Here's how the part is built. I have some questions about the finished solid (model axes, mm). A direction names the side the tool comes from. Round coordinates to 2 decimals unless told otherwise and drop trailing zeros. Loops run counter-clockwise (first coordinate to the right, second up) from the corner with the lowest first, then second, coordinate; pieces in that order, holes last. Notation, with made-up numbers: (82, 3.5) -> (141, 3.5) arc R29 ccw to (141, 36.5) -> close; hole circle Ø3 at (-39.75, 34). An arc over 180 degrees is marked (long way). Use CSV: the item, a comma, the result in double quotes. Start each with the question number.
Autodesk Inventor part; units mm, degrees
ref_plane "YZ Plane" through (0, 0, 0) normal (1, 0, 0) x (0, 1, 0)
ref_plane "XZ Plane" through (0, 0, 0) normal (0, 1, 0) x (-1, 0, 0)
ref_plane "XY Plane" through (0, 0, 0) normal (0, 0, 1) x (1, 0, 0)
sketch "Sketch1" plane through (0, 0, 0) normal (0, 0, 1) x (1, 0, 0)
  line L0 (-95, -10) -> (95, -10)
  line L1 (95, -10) -> (95, 10)
  line L2 (95, 10) -> (-95, 10)
  line L3 (-95, 10) -> (-95, -10)
  line L4 (-95, -10) -> (95, 10) construction
  line L5 (95, -10) -> (-95, 10) construction
  line L6 (-133, 0) -> (133, 0) construction
  line L7 (-83, -5.5) -> (-6, -5.5)
  line L8 (-6, -5.5) -> (-6, 5.5)
  line L9 (-6, 5.5) -> (-83, 5.5)
  line L10 (-83, 5.5) -> (-83, -5.5)
  line L11 (-83, -5.5) -> (-6, 5.5) construction
  line L12 (-6, -5.5) -> (-83, 5.5) construction
  line L13 (0, 14.2899) -> (0, -14.2899) construction
  line L14 (83, -5.5) -> (6, -5.5)
  line L15 (6, -5.5) -> (6, 5.5)
  line L16 (6, 5.5) -> (83, 5.5)
  line L17 (83, 5.5) -> (83, -5.5)
  line L18 (83, -5.5) -> (6, 5.5) construction
  line L19 (6, -5.5) -> (83, 5.5) construction
  circle A0 centre (-89, 0) radius 2.75
  circle A1 centre (0, 0) radius 2.75
  circle A2 centre (89, 0) radius 2.75
  line L20 (-83, 5.5) -> (-73, 5.5)
  line L21 (-73, 5.5) -> (-73, -5.5)
  line L22 (-73, -5.5) -> (-83, -5.5)
  line L23 (-83, -5.5) -> (-83, 5.5)
  line L24 (-6, 5.5) -> (-16, 5.5)
  line L25 (-16, 5.5) -> (-16, -5.5)
  line L26 (-16, -5.5) -> (-6, -5.5)
  line L27 (-6, -5.5) -> (-6, 5.5)
  line L28 (16, 5.5) -> (16, -5.5)
  line L29 (73, 5.5) -> (73, -5.5)
  line L30 (6, 10) -> (6, 5.4904)
  line L31 (6, 5.4904) -> (6, -10)
  point P0 (-44.5, 0)
  point P1 (44.5, 0)
  point P2 (73, -5.5)
  point P3 (73, 5.5)
  point P4 (-73, 5.5)
  point P5 (6, -5.5)
  dimension "d0" = 190
  dimension "d1" = 20
  dimension "d2" = 11
  dimension "d3" = 12
  dimension "d4" = 6
  dimension "d5" = 5.5
  dimension "d6" = 6
  dimension "d7" = 5.5
  dimension "d11" = 10
  dimension "d12" = 10
extrude "Extrusion1" add sketch "Sketch1" along normal blind 3 contours L3 L2 L30 L15 L31 L0 | L21 L9 L25 L7
fillet "Fillet1" radius 1 4 edges at (-95, -10, 1.5) (-95, 10, 1.5) (6, 10, 1.5) (6, -10, 1.5)
sketch "Sketch2" plane through (0, 0, 3) normal (0, 0, 1) x (1, 0, 0)
  line L0 (-16, 5.5) -> (-6, 5.5)
  line L1 (-6, 5.5) -> (-6, -5.5)
  line L2 (-6, -5.5) -> (-16, -5.5)
  line L3 (-16, -5.5) -> (-16, 5.5)
  circle A0 centre (-89, 0) radius 2.75
  circle A1 centre (0, 0) radius 2.75
  arc A2 (5, -10) -> (6, -9) centre (5, -9) ccw
  line L4 (6, -9) -> (6, 9)
  arc A3 (6, 9) -> (5, 10) centre (5, 9) ccw
  line L5 (5, 10) -> (-94, 10)
  arc A4 (-94, 10) -> (-95, 9) centre (-94, 9) ccw
  line L6 (-95, 9) -> (-95, -9)
  arc A5 (-95, -9) -> (-94, -10) centre (-94, -9) ccw
  line L7 (-94, -10) -> (5, -10)
  line L8 (-73, 5.5) -> (-73, -5.5)
  line L9 (-73, -5.5) -> (-83, -5.5)
  line L10 (-83, -5.5) -> (-83, 5.5)
  line L11 (-83, 5.5) -> (-73, 5.5)
equation "\"d6\" = 0.5 * d3"
equation "\"d7\" = d5"
equation "\"d12\" = d11"
properties part number "LED_Holder_BackTop"
Q1. I want a section at C-C, the plane x = -9.5. List the corners of the cut face in (y, z) for me.
Q2. I need wall thicknesses on line 1 along X through (y, z) = (-4, 1.6); line 2 along Y through (x, z) = (-76.5, 0.2); line 3 along Y through (x, z) = (-89, 1.95). Which ranges of each line are inside material? Lowest first, please.
Q3. If we mould it in two halves opening along X, with no side actions, what happens to faces 3 (the cylindrical face through (-91.747, -0.121, 1.479)), 4 (the flat face through (-95, 0, 1)), 5 (the flat face through (6, 0, 1))? For each: pulls with the +X half, pulls with the -X half, needs draft (parallel to the pull), parting line crosses it, or undercut.
Q4. I want a section at A-A, the plane x = -89. List the corners of the cut face in (y, z) for me.
Q5. I want a section at B-B, the plane y = 0. List the corners of the cut face in (x, z) for me.
Q6. For faces 1 (the flat face through (-45, 0, 3)), 2 (the flat face through (-11, 5.5, 1)), which set-ups out of +Z, -Z, +X, -X, +Y, -Y let a thin tool reach every point of the face, with its end or its side?
Values found:
1,outline,"(-10, 0) -> (-5.5, 0) -> (-5.5, 3) -> (-10, 3) -> close; (5.5, 0) -> (10, 0) -> (10, 3) -> (5.5, 3) -> close"
2,line 1,"-95 to -83, -73 to -16, -6 to 6"
2,line 2,"-10 to -5.5, 5.5 to 10"
2,line 3,"-10 to -2.75, 2.75 to 10"
3,face 3,"undercut"
3,face 4,"pulls with the -X half"
3,face 5,"pulls with the +X half"
4,outline,"(-10, 0) -> (-2.75, 0) -> (-2.75, 3) -> (-10, 3) -> close; (2.75, 0) -> (10, 0) -> (10, 3) -> (2.75, 3) -> close"
5,outline,"(-95, 0) -> (-91.75, 0) -> (-91.75, 3) -> (-95, 3) -> close; (-86.25, 0) -> (-83, 0) -> (-83, 3) -> (-86.25, 3) -> close; (-73, 0) -> (-16, 0) -> (-16, 3) -> (-73, 3) -> close; (-6, 0) -> (-2.75, 0) -> (-2.75, 3) -> (-6, 3) -> close; (2.75, 0) -> (6, 0) -> (6, 3) -> (2.75, 3) -> close"
6,face 1,"+Z, +X, -X, +Y, -Y"
6,face 2,"+Z, -Z"
